Autodesk Inventor part; units mm, degrees
ref_plane "YZ Plane" through (0, 0, 0) normal (1, 0, 0) x (0, 1, 0)
ref_plane "XZ Plane" through (0, 0, 0) normal (0, 1, 0) x (-1, 0, 0)
ref_plane "XY Plane" through (0, 0, 0) normal (0, 0, 1) x (1, 0, 0)
sketch "Sketch1" plane through (0, 0, 0) normal (0, 0, 1) x (1, 0, 0)
  point P0 (0, 0)
sketch "Sketch2" plane through (0, 0, 0) normal (0, 0, 1) x (1, 0, 0)
  line L0 (-9.8946, 8.2346) -> (40.1054, 8.2346)
  line L1 (40.1054, 8.2346) -> (40.1054, -51.7654)
  line L2 (40.1054, -51.7654) -> (-9.8946, -51.7654)
  line L3 (-9.8946, -51.7654) -> (-9.8946, 8.2346)
  point P0 (0, 0)
  dimension "d0" = 50
  dimension "d1" = 60
extrude "Extrusion1" add sketch "Sketch2" along normal blind 30
sketch "Sketch3" plane through (-9.8946, 8.2346, 0) normal (0, 1, 0) x (1, 0, 0)
  line L0 (2.3069, -21.5805) -> (5.2632, -21.5805)
  line L1 (5.2632, -21.5805) -> (5.2632, -7.9818)
  line L2 (5.2632, -7.9818) -> (2.3069, -7.9818)
  line L3 (2.3069, -7.9818) -> (2.3069, -21.5805)
  line L4 (43.8913, -21.5805) -> (47.0446, -21.5805)
  line L5 (47.0446, -21.5805) -> (47.0446, -7.9818)
  line L6 (47.0446, -7.9818) -> (43.8913, -7.9818)
  line L7 (43.8913, -7.9818) -> (43.8913, -21.5805)
  point P0 (9.8946, 0)
extrude "Extrusion2" add sketch "Sketch3" along normal blind 3.5
sketch "Sketch4" plane through (-9.8946, 8.2346, 0) normal (0, 1, 0) x (1, 0, 0)
  circle A0 centre (12.2632, -15) radius 3.5
  line L0 (50, -30) -> (0, -30)
  circle A1 centre (36.8913, -14.7812) radius 3.5
  line L1 (5.2632, -21.5805) -> (5.2632, -7.9818)
  line L2 (43.8913, -7.9818) -> (43.8913, -21.5805)
  point P0 (9.8946, 0)
  point P1 (5.2632, -14.7812)
  point P2 (43.8913, -14.7812)
  dimension "d6" = 15
  dimension "d7" = 7
  dimension "d8" = 7
  dimension "d9" = 7
  dimension "d10" = 24.6281
  dimension "d11" = 7
extrude "Extrusion3" add sketch "Sketch4" along normal blind 3.5
properties part number "battery"
Geometry check sheet. Reference: the model listing, model coordinates, mm. A direction names the side the tool comes from. Coordinates: 2 decimals unless noted, no trailing zeros. Order: outer loops, then holes, each group sorted by start corner. A loop starts at its lowest first (then second) coordinate and runs counter-clockwise, first axis right, second up. Notation, with made-up numbers: (-35, 3.5) -> (13, 3.5) arc R23 cw to (13, 33.5) -> close; hole circle Ø1 at (63, 57). An arc over 180 degrees is marked (long way). Use a Markdown table: item, result. Add a question column.
1. Set-up check for faces 5 (the face through (1.61, 9.96, 11.583)), 6 (the face through (-4.631, 10, 15)), 7 (the face through (36, 10, 21.58)): record each of +Z, -Z, +X, -X, +Y, -Y from which the full face is reachable in a straight line by a thin tool's end or side.
2. Material ranges on L1, parallel to Y at x = 13.5, z = 14.75, recorded low to high.
3. Go/stop test with flat-tipped pins: pin 1 Ø3 at (y, z) = (11, 12) entering from -X; pin 2 Ø3 at (y, z) = (10.5, 15) entering from +X; pin 3 Ø3 at (x, z) = (28, 6.5) entering from +Y. Record where each tip stops, or that it passes through.
4. Mould release check, pull along X, two halves, no side actions. Record for faces 1 (the face through (-7.588, 10, 15)), 2 (the face through (37.15, 10, 15)), 3 (the face through (36, 10, 7.982)), 4 (the face through (33.997, 10, 15)): pulls with the +X half, pulls with the -X half, needs draft (parallel to the pull), parting line crosses it, or undercut.
5. Cross-section at A-A (x = 35.5). Enter the section's corners in (y, z), and give its area (3 significant figures).
6. Cross-section at B-B (z = 2.75). Enter the section's corners in (x, y).
Filled sheet:
| question | item | result |
|---|---|---|
| 1 | face 5 | +Y |
| 1 | face 6 | +Z, -Z, +Y |
| 1 | face 7 | +Z, +X, -X, +Y |
| 2 | L1 | -51.77 to 8.23 |
| 3 | pin 1 | x = -7.59 |
| 3 | pin 2 | x = 37.15 |
| 3 | pin 3 | y = 8.23 |
| 4 | face 1 | pulls with the -X half |
| 4 | face 2 | pulls with the +X half |
| 4 | face 3 | needs draft |
| 4 | face 4 | undercut |
| 5 | outline | (-51.77, 0) -> (8.23, 0) -> (8.23, 7.98) -> (11.73, 7.98) -> (11.73, 21.58) -> (8.23, 21.58) -> (8.23, 30) -> (-51.77, 30) -> close |
| 5 | area | 1,850 mm2 |
| 6 | outline | (-9.89, -51.77) -> (40.11, -51.77) -> (40.11, 8.23) -> (-9.89, 8.23) -> close |
